from build123d import *

# Parameters (mm, degrees)
EXTRUDE_1_DEPTH = 150
EXTRUDE_START   = -49.25
EXTRUDE_2_DEPTH = 51.5
FILLET_1_R      = 0.1
FILLET_2_R      = 0.2


with BuildPart() as part:
    # 草图1 → 凸台-拉伸1 (new body)
    with BuildSketch(Plane.XY):
        Polygon((0, 0), (0, 31), (-2, 31), (-2, 0.828427125), (-13.435028843, -10.606601718), (-10.606601718, -10.606601718), align=None)
    extrude(amount=EXTRUDE_1_DEPTH)

    # 草图3 → 凸台-拉伸2 (add)
    with BuildSketch(Plane.XY.offset(150).offset(EXTRUDE_START)):
        with BuildLine():
            Line((0, 9.5), (0, 8))
            Line((0, 8), (0.677124344, 8))
            ThreePointArc((0.677124344, 8), (1.088161527, 7.719957697), (1.555590279, 7.55))
            Line((1.555590279, 7.55), (2.5, 7.55))
            Line((2.5, 7.55), (2.5, 8.056624327))
            Line((2.5, 8.056624327), (0, 9.5))
        make_face()
    extrude_2 = extrude(amount=-EXTRUDE_2_DEPTH)

    # 镜向1: 凸台-拉伸2 across plane
    add(extrude_2.mirror(Plane.ZX.offset(9.5)))

    # 圆角1
    fillet_1_edges = [part.edges().sort_by_distance(p)[0] for p in [
        (2.5, 7.803312164, 49.25),
        (2.5, 8.056624327, 75),
        (2.5, 7.55, 75),
        (2.5, 7.803312164, 100.75),
        (2.5, 10.943375673, 75),
        (2.5, 11.196687836, 100.75),
        (2.5, 11.45, 75),
        (2.5, 11.196687836, 49.25),
    ]]
    fillet(fillet_1_edges, radius=FILLET_1_R)

    # 圆角2
    fillet_2_edges = [part.edges().sort_by_distance(p)[0] for p in [
        (-1, 31, 150),
        (-10.606601718, -10.606601718, 75),
        (-13.435028843, -10.606601718, 75),
        (-2, 0.828427125, 75),
        (-2, 31, 75),
        (0, 31, 75),
        (0, 0, 75),
        (-2, 15.914213562, 150),
        (-7.717514421, -4.889087297, 150),
        (-12.02081528, -10.606601718, 150),
        (-5.303300859, -5.303300859, 150),
        (-12.02081528, -10.606601718, 0),
        (-7.717514421, -4.889087297, 0),
        (-2, 15.914213562, 0),
        (0, 15.5, 150),
        (-1, 31, 0),
        (0, 15.5, 0),
        (-5.303300859, -5.303300859, 0),
    ]]
    fillet(fillet_2_edges, radius=FILLET_2_R)


solid = part.part
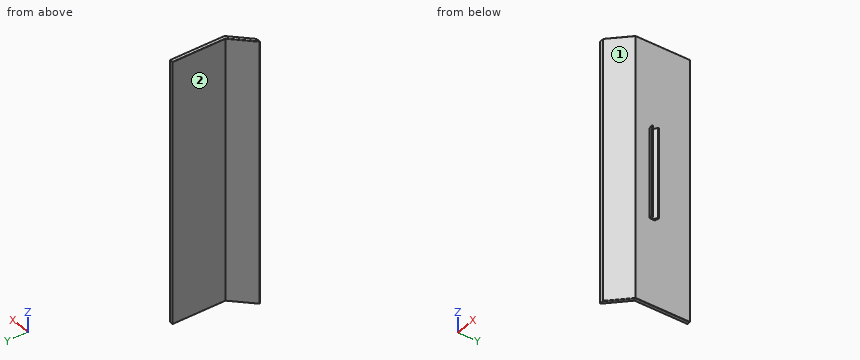
For this review, take the finished solid that the model builds, in its own axes (mm). Face numbers are marked on the shaded views. A direction names the side the tool comes from. Round coordinates to 2 decimals unless told otherwise and drop trailing zeros. Loops run counter-clockwise (first coordinate to the right, second up) from the corner with the lowest first, then second, coordinate; pieces in that order, holes last. Notation, with made-up numbers: (63.5, 64.25) - (78.5, 64.25) arc R19 ccw to (78.5, 77.25) - close; hole circle Ø2 at (61, -12.75). An arc over 180 degrees is marked (long way). Use one line per item in the form item = value.
Item 1: Consider section A-A on z = 16.5. Write out the cut boundary in (x, y), then the cut area to 3 significant figures.
Answers:
outline = (-13.09, -10.27) arc R0.2 ccw to (-12.95, -10.61) - (-10.69, -10.61) arc R0.2 ccw to (-10.55, -10.55) - (-0.06, -0.06) arc R0.2 ccw to (0, 0.08) - (0, 30.8) arc R0.2 ccw to (-0.2, 31) - (-1.8, 31) arc R0.2 ccw to (-2, 30.8) - (-2, 0.91) arc R0.2 cw to (-2.06, 0.77) - close
area = 92.3 mm^2
Item 2: Tool access review of the marked faces 1 and 2: name each direction out of +Z, -Z, +X, -X, +Y, -Y from which nothing blocks a thin tool from reaching the whole face with its end or side.
Answers:
face_1 = +Z, -Z, +X, -Y
face_2 = +Z, -Z, -X, +Y
Item 3: Consider section C-C on z = 70. Write out the cut boundary in (x, y).
Answers:
outline = (-13.09, -10.27) arc R0.2 ccw to (-12.95, -10.61) - (-10.69, -10.61) arc R0.2 ccw to (-10.55, -10.55) - (-0.06, -0.06) arc R0.2 ccw to (0, 0.08) - (0, 8) - (0.68, 8) arc R2 ccw to (1.56, 7.55) - (2.4, 7.55) arc R0.1 ccw to (2.5, 7.65) - (2.5, 8) arc R0.1 ccw to (2.45, 8.09) - (0, 9.5) - (2.45, 10.91) arc R0.1 ccw to (2.5, 11) - (2.5, 11.35) arc R0.1 ccw to (2.4, 11.45) - (1.56, 11.45) arc R2 ccw to (0.68, 11) - (0, 11) - (0, 30.8) arc R0.2 ccw to (-0.2, 31) - (-1.8, 31) arc R0.2 ccw to (-2, 30.8) - (-2, 0.91) arc R0.2 cw to (-2.06, 0.77) - close
Item 4: Consider section B-B on y = 14.5. Write out the cut boundary in (x, z).
Answers:
outline = (-2, 0.2) arc R0.2 ccw to (-1.8, 0) - (-0.2, 0) arc R0.2 ccw to (0, 0.2) - (0, 149.8) arc R0.2 ccw to (-0.2, 150) - (-1.8, 150) arc R0.2 ccw to (-2, 149.8) - close
Item 5: For line 1 (X direction, y = 28, z = 109); line 2 (Y direction, x = -5, z = 88); line 3 (Y direction, x = -1.25, z = 94), list the stretches that pass through material, from the lowest coordinate up.
Answers:
line_1 = -2 to 0
line_2 = -5 to -2.17
line_3 = -1.25 to 31
Item 6: Clearance check with flat-ended pins moving along their axes: P1, Ø6, axis at x = -1, z = 110.5, coming from the -Y side; P2, Ø1.6, axis at x = 1.5, y = 8.5, coming from the -Z side; P3, Ø5, axis at x = -3.5, z = 95, coming from the -Y side. State where each tip first meets the part, or that it passes through.
Answers:
P1 = -4
P2 = 49.25
P3 = -6
